Check sheet for the drawn part. Datum: minimum x, y, z corner. Units: mm. Give positions to 0.01 mm unless a question says otherwise; leave off trailing zeros. Order: outer loops, then holes, each group sorted by start corner. A loop starts at its lowest first (then second) coordinate and runs counter-clockwise, first axis right, second up.
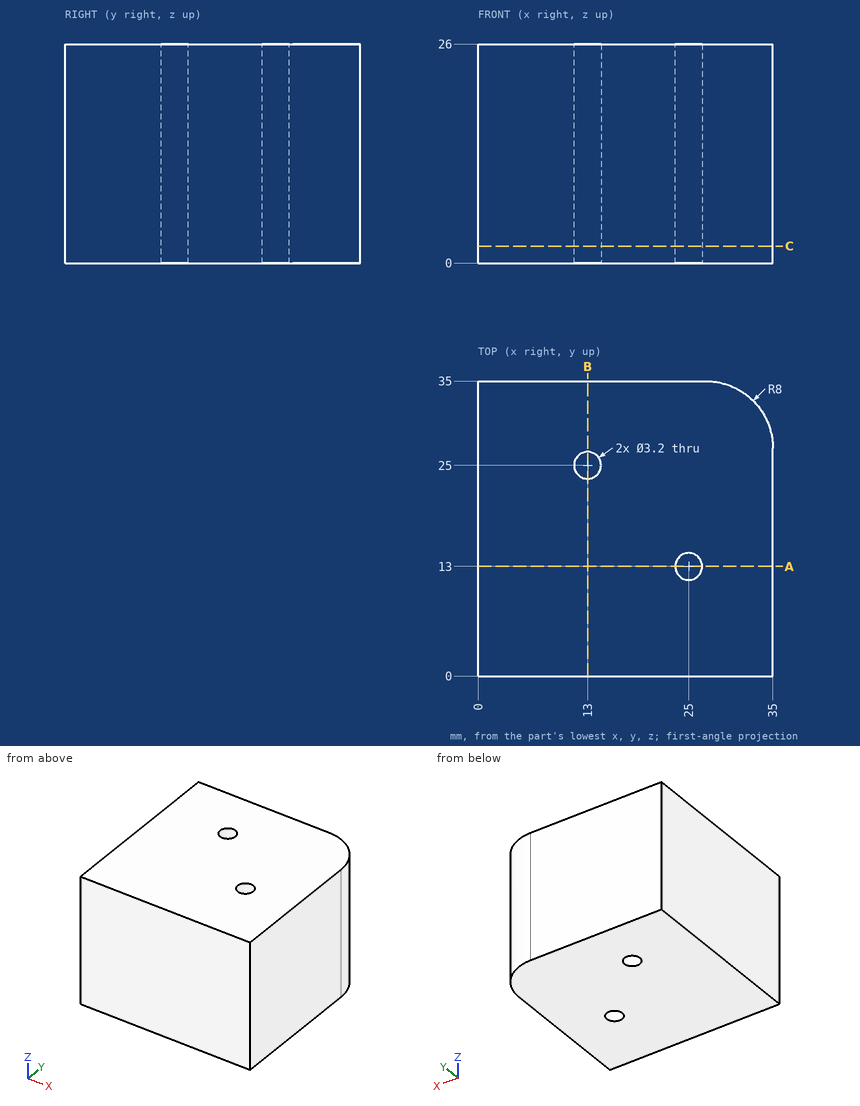
Item 1: Gauge pin test, flat end, axial feed: pin 1 (3 mm diameter, centred on x = 25, y = 13, fed in from -Z). Record the tip position at first contact, or that the pin passes through.
Reported:
pin 1: passes through
Item 2: Sectioned sample at C-C (z = 2). Enter the section's corners in (x, y), and give its area (3 significant figures).
Reported:
outline: (0, 0) - (35, 0) - (35, 27) arc R8 ccw to (27, 35) - (0, 35) - close; hole circle Ø3.2 at (13, 25); hole circle Ø3.2 at (25, 13)
area: 1,200 mm2
Item 3: Sectioned sample at A-A (y = 13). Enter the section's corners in (x, z), and give its area (3 significant figures).
Reported:
outline: (0, 0) - (23.4, 0) - (23.4, 26) - (0, 26) - close; (26.6, 0) - (35, 0) - (35, 26) - (26.6, 26) - close
area: 827 mm2
Item 4: Scan lines: L1, parallel to Y at x = 13, z = 5.5; L2, parallel to Y at x = 25, z = 6.5; L3, parallel to X at y = 24.5, z = 7.25. Record each from-to range of solid material in increasing order.
Reported:
L1: y = 0 to 23.4, 26.6 to 35
L2: y = 0 to 11.4, 14.6 to 35
L3: x = 0 to 11.48, 14.52 to 35
